Model file for the job. Use its own axes, mm. Face numbers are marked on the shaded views. A direction names the side the tool comes from. Round coordinates to 2 decimals unless told otherwise and drop trailing zeros. Loops run counter-clockwise (first coordinate to the right, second up) from the corner with the lowest first, then second, coordinate; pieces in that order, holes last. Notation, with made-up numbers: (43, -23.5) -> (74, -23.5) arc R35 cw to (74, 11.5) -> close; hole circle Ø1 at (29, 79). An arc over 180 degrees is marked (long way). Use a Markdown table: item, result.
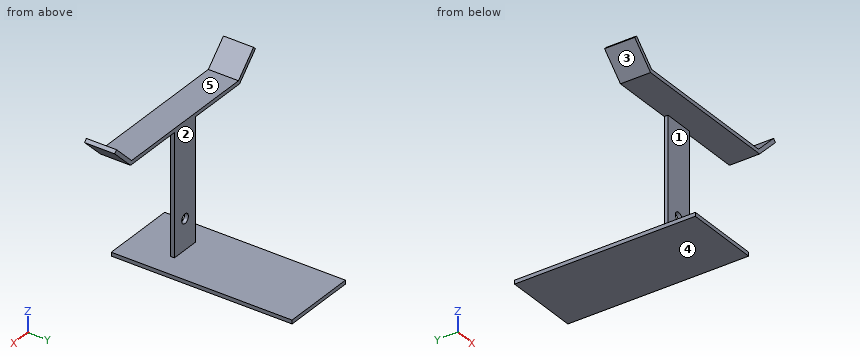
from build123d import *

# Parameters (mm, degrees)
F0_W     = 127
F0_H     = 304.8
F1_DEPTH = 6.35
F2_W     = 50.8
F2_H     = 6.35
F3_DEPTH = 203.2
F5_D     = 15.875
F7_DEPTH = 50.8


with BuildPart() as f1:
    # F0 (on Top) → F1 (new body)
    with BuildSketch(Plane.XY):
        Rectangle(F0_W, F0_H)
    extrude(amount=-F1_DEPTH)

    # F2 (on face) → F3 (join)
    with BuildSketch(Plane.XY):
        with Locations((0, -76.2)):
            Rectangle(F2_W, F2_H)
    extrude(amount=F3_DEPTH)

    # F5 (through all)
    with Locations(Plane.XZ.offset(79.375)):
        with Locations((0, 50.8)):
            Hole(F5_D / 2)

    # F6 (on face) → F7 (join)
    with BuildSketch(Plane(origin=(0, -73.025, 0), x_dir=(-1, 0, 0), z_dir=(0, 1, 0))):
        Polygon((-129.630256, 203.2), (-127, 203.2), (127, 203.2), (129.630256, 203.2), (167.411153, 240.980896), (162.921024, 245.471024), (127, 209.55), (-127, 209.55), (-162.921024, 245.471024), (-167.411153, 240.980896), align=None)
    extrude(amount=-F7_DEPTH)


solid = f1.part
Q1. Band-saw the part on D-D, the plane y = 91.5. Give the cut face in (x, z).
Results list:
| item | result |
|---|---|
| outline | (-63.5, -6.35) -> (63.5, -6.35) -> (63.5, 0) -> (-63.5, 0) -> close |
Q2. Drill centre lines: L1, parallel to Z at x = 0, y = -75; L2, parallel to Z at x = 15.5, y = -87; L3, parallel to X at y = -77, z = 50. Where is each one in solid material? Low to high. Write a range as from..to.
Results list:
| item | result |
|---|---|
| L1 | z = -6.35..42.86, 58.74..209.55 |
| L2 | z = -6.35..0, 203.2..209.55 |
| L3 | x = -25.4..-7.9, 7.9..25.4 |
Q3. Pull direction Z, two halves, no side cores. Call the marked faces 1, 2 and 3: released by +Z, released by -Z, zero draft, split by the parting line, or undercut.
Results list:
| item | result |
|---|---|
| face 1 | undercut |
| face 2 | zero draft |
| face 3 | released by -Z |
Q4. Band-saw the part on B-B, the plane z = 50.8. Give the cut face in (x, y) (1 decimal), plus the area to 3 significant figures.
Results list:
| item | result |
|---|---|
| outline | (-25.4, -79.4) -> (-7.9, -79.4) -> (-7.9, -73) -> (-25.4, -73) -> close; (7.9, -79.4) -> (25.4, -79.4) -> (25.4, -73) -> (7.9, -73) -> close |
| area | 222 mm² |
Q5. Flat gauge pins, fed straight in: pin 1 (5 mm diameter, centred on y = 8, z = -4.5, fed in from +X); pin 2 (1.9 mm diameter, centred on y = -77, z = 85, fed in from -X); pin 3 (1 mm diameter, centred on x = -19.5, y = -108.5, fed in from +Z). Where does each tip first touch, or does it go through?
Results list:
| item | result |
|---|---|
| pin 1 | stops at x = 63.5 |
| pin 2 | stops at x = -25.4 |
| pin 3 | stops at z = 209.55 |
Q6. Band-saw the part on C-C, the plane z = 228.5. Give the cut face in (x, y) (3 decimals).
Results list:
| item | result |
|---|---|
| outline | (-154.93, -123.825) -> (-145.95, -123.825) -> (-145.95, -73.025) -> (-154.93, -73.025) -> close; (145.95, -123.825) -> (154.93, -123.825) -> (154.93, -73.025) -> (145.95, -73.025) -> close |
Q7. Tool access for the marked faces 4 and 5: list every direction of +Z, -Z, +X, -X, +Y, -Y with a clear straight run to the whole face (end or side of a thin tool).
Results list:
| item | result |
|---|---|
| face 4 | -Z, +X, -X, +Y, -Y |
| face 5 | +Z, +Y, -Y |
